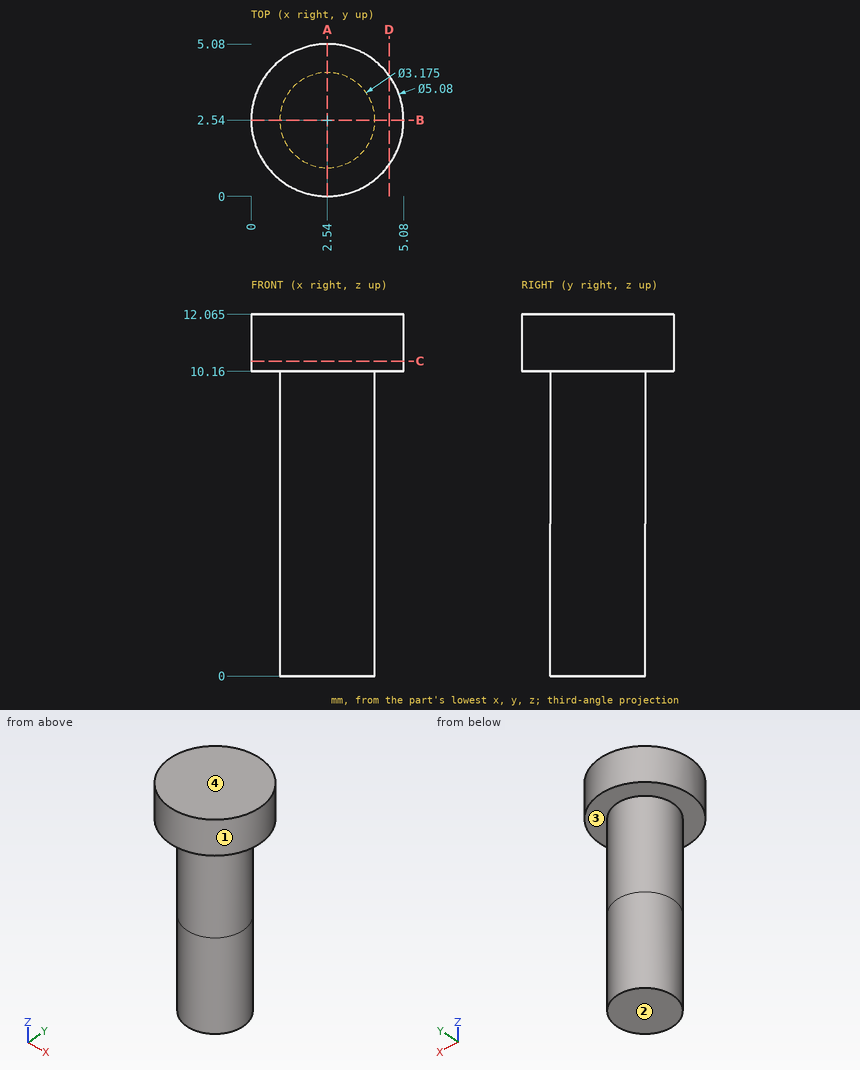
Print and shaded views of the part. All mm, measured from the part's lowest x, y and z. A direction names the side the tool comes from. Give positions to 0.01 mm unless a question says otherwise; leave off trailing zeros. Loops run counter-clockwise (first coordinate to the right, second up) from the corner with the lowest first, then second, coordinate; pieces in that order, holes last.
1) Tool access for the marked faces 3 and 4: list every direction of +Z, -Z, +X, -X, +Y, -Y with a clear straight run to the whole face (end or side of a thin tool).
2) Pull direction X, two halves, no side cores. Call the marked faces 1 and 2: +X half, -X half, draft (parallel to the pull), parting line (faces both ways), or undercut.
3) Saw through at C-C (z = 10.5). Write the cut outline in (x, y).
4) Wall check: line 1 (Z direction, x = 1.45, y = 1) (3 decimals); line 2 (Y direction, x = 2.45, z = 11.25); line 3 (X direction, y = 3.45, z = 10.75). Give the ranges that are in metal, low to high.
5) Saw through at D-D (x = 4.6). Write the cut outline in (y, z) (3 decimals).
6) Saw through at A-A (x = 2.54). Write the cut outline in (y, z) (1 decimal).
7) Flat gauge pin, fed straight in: pin 1 Ø1.5 at (y, z) = (2, 6.5) entering from -X. Where does the tip first touch, or does it go through?
Answer block:
1. face 3: -Z
1. face 4: +Z, +X, -X, +Y, -Y
2. face 1: parting line
2. face 2: draft
3. outline: circle Ø5.08 at (2.54, 2.54)
4. line 1: z = 10.16 to 12.065
4. line 2: y = 0 to 5.08
4. line 3: x = 0.17 to 4.91
5. outline: (1.054, 10.16) - (4.026, 10.16) - (4.026, 12.065) - (1.054, 12.065) - close
6. outline: (0, 10.2) - (1, 10.2) - (1, 0) - (4.1, 0) - (4.1, 10.2) - (5.1, 10.2) - (5.1, 12.1) - (0, 12.1) - close
7. pin 1: stops at x = 0.95
